Part model, mm, in its own coordinate system. Round coordinates to 2 decimals unless told otherwise and drop trailing zeros. Loops run counter-clockwise (first coordinate to the right, second up) from the corner with the lowest first, then second, coordinate; pieces in that order, holes last. Notation, with made-up numbers: (19, 85) - (59, 85) arc R19 ccw to (59, 98) - close; hole circle Ø4 at (21, 62.5). An arc over 180 degrees is marked (long way). Write each question's results on one line, items separated by ' | '. Start each with the question number.
(1) Flat gauge pins, fed straight in: P1, Ø1, axis at y = -33, z = 2, coming from the -X side; P2, Ø1.5, axis at x = -11, z = 2, coming from the -Y side; P3, Ø1, axis at y = -77, z = 4, coming from the +X side. Where does each tip first touch, or does it go through?
(2) Cut at A-A, the plane x = -73.5. List the corners of the cut face in (y, z), then the cut area to 3 significant figures.
(3) Cut at B-B, the plane y = -77. List the corners of the cut face in (x, z), then the cut area to 3 significant figures.
(4) Drill centre lines: L1, parallel to X at y = -115.5, z = 1.1; L2, parallel to X at y = -134.5, z = 2.1; L3, parallel to Y at x = -17.5, z = 0.4. Where is each one in solid material? Low to high.
(5) Cut at C-C, the plane z = 0.85. Give the number of separate pieces and of enclosed holes in the cut face, then the cut area to 3 significant figures.
(6) Mould opens along X. For faces 1 (the face through (-1, 11, 0)), 2 (the face through (-122.85, 128.373, 2.465)) say: released by +X, released by -X, zero draft, split by the parting line, or undercut.
from build123d import *

# Parameters (mm, degrees)
EXTRUDE_246_DEPTH       = 5
EXTRUDE_363_DEPTH       = 5
SKETCH_3_R              = 20
EXTRUDE_433_DEPTH       = 5
SKETCH_4_R              = 4
SKETCH_4_R_2            = 1.6
SKETCH_4_R_3            = 1.1
CUT_EXTRUDE_574_DEPTH   = 5
SKETCH_5_R              = 1.1
CUT_EXTRUDE_636_DEPTH   = 5
SKETCH_7_R              = 1.65
CUT_EXTRUDE_M3_DEPTH    = 5
SKETCH_8_R              = 1.65
PIXHAWK_M3_54X60_DEPTH  = 5
SKETCH_9_W              = 10
SKETCH_9_H              = 26.682090866
SKETCH_9_W_2            = 26.682090866
SKETCH_9_H_2            = 10
CUT_EXTRUDE_20X12_DEPTH = 5


with BuildPart() as part:
    # 草图1 → Extrude 246 (new body)
    with BuildSketch(Plane.XY):
        Polygon((50, 25), (25, 50), (-25, 50), (-50, 25), (-50, -25), (-25, -50), (25, -50), (50, -25), align=None)
    extrude(amount=EXTRUDE_246_DEPTH)

    # 草图2 → Extrude 363 (add)
    with BuildSketch(Plane.XY):
        Polygon((14.849242405, 30.405591591), (120.050252532, 135.606601718), (135.606601718, 120.050252532), (30.405591591, 14.849242405), align=None)
        Polygon((-30.405591591, 14.849242405), (-135.606601718, 120.050252532), (-120.050252532, 135.606601718), (-14.849242405, 30.405591591), align=None)
        Polygon((-14.849242405, -30.405591591), (-120.050252532, -135.606601718), (-135.606601718, -120.050252532), (-30.405591591, -14.849242405), align=None)
        Polygon((30.405591591, -14.849242405), (135.606601718, -120.050252532), (120.050252532, -135.606601718), (14.849242405, -30.405591591), align=None)
    extrude(amount=EXTRUDE_363_DEPTH)

    # 草图3 → Extrude 433 (add)
    with BuildSketch(Plane.XY):
        with Locations((-125, -125)):
            Circle(SKETCH_3_R)
        with Locations((-125, 125)):
            Circle(SKETCH_3_R)
        with Locations((125, -125)):
            Circle(SKETCH_3_R)
        with Locations((125, 125)):
            Circle(SKETCH_3_R)
    extrude(amount=EXTRUDE_433_DEPTH)

    # 草图4 → Cut-Extrude 574 (cut)
    with BuildSketch(Plane.XY):
        with Locations((-125, -125)):
            Circle(SKETCH_4_R)
        with Locations((-35, -35)):
            Circle(SKETCH_4_R_2)
        with Locations((-8, -40)):
            Circle(SKETCH_4_R_3)
        with Locations((-125, 125)):
            Circle(SKETCH_4_R)
        with Locations((-35, 35)):
            Circle(SKETCH_4_R_2)
        with Locations((-8, 40)):
            Circle(SKETCH_4_R_3)
        with Locations((125, -125)):
            Circle(SKETCH_4_R)
        with Locations((35, -35)):
            Circle(SKETCH_4_R_2)
        with Locations((8, -40)):
            Circle(SKETCH_4_R_3)
        with Locations((125, 125)):
            Circle(SKETCH_4_R)
        with Locations((35, 35)):
            Circle(SKETCH_4_R_2)
        with Locations((8, 40)):
            Circle(SKETCH_4_R_3)
        with Locations((-15.25, -15.25)):
            Circle(SKETCH_4_R_2)
        with Locations((-15.25, 15.25)):
            Circle(SKETCH_4_R_2)
        with Locations((15.25, -15.25)):
            Circle(SKETCH_4_R_2)
        with Locations((15.25, 15.25)):
            Circle(SKETCH_4_R_2)
        with Locations((-10, -10)):
            Circle(SKETCH_4_R_2)
        with Locations((-10, 10)):
            Circle(SKETCH_4_R_2)
        with Locations((10, -10)):
            Circle(SKETCH_4_R_2)
        with Locations((10, 10)):
            Circle(SKETCH_4_R_2)
        with Locations((-134.5, -125)):
            Circle(SKETCH_4_R_2)
        with Locations((-125, -134.5)):
            Circle(SKETCH_4_R_2)
        with Locations((-115.5, -125)):
            Circle(SKETCH_4_R_2)
        with Locations((-125, -115.5)):
            Circle(SKETCH_4_R_2)
        with Locations((-134.5, 125)):
            Circle(SKETCH_4_R_2)
        with Locations((-125, 115.5)):
            Circle(SKETCH_4_R_2)
        with Locations((-115.5, 125)):
            Circle(SKETCH_4_R_2)
        with Locations((-125, 134.5)):
            Circle(SKETCH_4_R_2)
        with Locations((115.5, -125)):
            Circle(SKETCH_4_R_2)
        with Locations((125, -134.5)):
            Circle(SKETCH_4_R_2)
        with Locations((134.5, -125)):
            Circle(SKETCH_4_R_2)
        with Locations((125, -115.5)):
            Circle(SKETCH_4_R_2)
        with Locations((115.5, 125)):
            Circle(SKETCH_4_R_2)
        with Locations((125, 115.5)):
            Circle(SKETCH_4_R_2)
        with Locations((134.5, 125)):
            Circle(SKETCH_4_R_2)
        with Locations((125, 134.5)):
            Circle(SKETCH_4_R_2)
    extrude(amount=CUT_EXTRUDE_574_DEPTH, mode=Mode.SUBTRACT)

    # 草图5 → Cut-Extrude 636 (cut)
    with BuildSketch(Plane.XY):
        with Locations((-40, -24)):
            Circle(SKETCH_5_R)
        with Locations((-40, 24)):
            Circle(SKETCH_5_R)
        with Locations((40, -24)):
            Circle(SKETCH_5_R)
        with Locations((40, 24)):
            Circle(SKETCH_5_R)
    extrude(amount=CUT_EXTRUDE_636_DEPTH, mode=Mode.SUBTRACT)

    # 草图7 → 托板机臂中线四孔_M3 (cut)
    with BuildSketch(Plane.XY):
        with Locations((-62, -62)):
            Circle(SKETCH_7_R)
        with Locations((-62, 62)):
            Circle(SKETCH_7_R)
        with Locations((62, -62)):
            Circle(SKETCH_7_R)
        with Locations((62, 62)):
            Circle(SKETCH_7_R)
    extrude(amount=CUT_EXTRUDE_M3_DEPTH, mode=Mode.SUBTRACT)

    # 草图8 → Pixhawk托板支柱四孔_M3_54x60 (cut)
    with BuildSketch(Plane.XY):
        with Locations((-27, -30)):
            Circle(SKETCH_8_R)
        with Locations((-27, 30)):
            Circle(SKETCH_8_R)
        with Locations((27, -30)):
            Circle(SKETCH_8_R)
        with Locations((27, 30)):
            Circle(SKETCH_8_R)
    extrude(amount=PIXHAWK_M3_54X60_DEPTH, mode=Mode.SUBTRACT)

    # 草图9 → 飞控至电调矩形走线孔_20x12 (cut)
    with BuildSketch(Plane.XY):
        with Locations((-30, 0)):
            Rectangle(SKETCH_9_W, SKETCH_9_H)
        with Locations((0, -30)):
            Rectangle(SKETCH_9_W_2, SKETCH_9_H_2)
        with Locations((30, 0)):
            Rectangle(SKETCH_9_W, SKETCH_9_H)
        with Locations((0, 30)):
            Rectangle(SKETCH_9_W_2, SKETCH_9_H_2)
    extrude(amount=CUT_EXTRUDE_20X12_DEPTH, mode=Mode.SUBTRACT)


solid = part.part
A:
1) P1: x = -49.06 | P2: y = -50 | P3: x = 93.06
2) outline: (-89.06, 0) - (-57.94, 0) - (-57.94, 5) - (-89.06, 5) - close; (57.94, 0) - (89.06, 0) - (89.06, 5) - (57.94, 5) - close | area: 311 mm2
3) outline: (-92.56, 0) - (-61.44, 0) - (-61.44, 5) - (-92.56, 5) - close; (61.44, 0) - (92.56, 0) - (92.56, 5) - (61.44, 5) - close | area: 311 mm2
4) L1: -142.6 to -126.6, -123.4 to -99.94, 99.94 to 123.4, 126.6 to 142.6 | L2: -142.6 to -126.6, -123.4 to -107.4, 107.4 to 123.4, 126.6 to 142.6 | L3: -50 to 50
5) separate pieces: 1 | enclosed holes: 52 | area: 21,400 mm2
6) face 1: zero draft | face 2: undercut
